from build123d import *

# Parameters (mm, degrees)
SKETCH1_W           = 900
SKETCH1_H           = 600
BOSS_EXTRUDE1_DEPTH = 5
SKETCH2_R           = 30
CUT_EXTRUDE2_DEPTH  = 10
SKETCH3_R           = 30
CUT_EXTRUDE3_DEPTH  = 10


with BuildPart() as part:
    # Sketch1 → Boss-Extrude1 (new body)
    with BuildSketch(Plane.XY):
        with Locations((25.545851528, 338.64628821)):
            Rectangle(SKETCH1_W, SKETCH1_H)
    extrude(amount=BOSS_EXTRUDE1_DEPTH)

    # Sketch2 → Cut-Extrude2 (cut)
    with BuildSketch(Plane(origin=(0, 0, 0), x_dir=(-1, 0, 0), z_dir=(0, 0, -1))):
        with Locations((-175.545851528, 535.128567936)):
            Circle(SKETCH2_R)
    extrude(amount=-CUT_EXTRUDE2_DEPTH, mode=Mode.SUBTRACT)

    # Sketch3 → Cut-Extrude3 (cut)
    with BuildSketch(Plane(origin=(0, 0, 0), x_dir=(-1, 0, 0), z_dir=(0, 0, -1))):
        with Locations((-175.545851528, 143.938114846)):
            Circle(SKETCH3_R)
    extrude(amount=-CUT_EXTRUDE3_DEPTH, mode=Mode.SUBTRACT)


solid = part.part
Can you work these out from the model? Positions are in its coordinate system, mm. Give positions to 0.01 mm unless a question says otherwise; leave off trailing zeros. Loops run counter-clockwise (first coordinate to the right, second up) from the corner with the lowest first, then second, coordinate; pieces in that order, holes last. Notation, with made-up numbers: (81, 71) -> (124, 71) arc R19 cw to (124, 84) -> close; hole circle Ø11 at (-12, -35.75). An arc over 180 degrees is marked (long way). Return JSON: item names as keys, results as strings.
Q1. I need wall thicknesses on probe 1 along X at (y, z) = (162, 2.6); probe 2 along X at (y, z) = (154, 0.85). Which ranges of each line are inside material? Lowest first, please.
Checks:
{"probe 1": "x = -424.45 to 151.59, 199.5 to 475.55", "probe 2": "x = -424.45 to 147.28, 203.81 to 475.55"}
Q2. I want a section at B-B, the plane y = 163.5. List the corners of the cut face in (x, z) for me.
Checks:
{"outline": "(-424.45, 0) -> (152.8, 0) -> (152.8, 5) -> (-424.45, 5) -> close; (198.29, 0) -> (475.55, 0) -> (475.55, 5) -> (198.29, 5) -> close"}
Q3. We'd pull the mould along X, two halves only. Please class faces 1 (the face through (19, 343, 0)), 2 (the face through (161.703, 508.513, 2.465)): released by +X, released by -X, zero draft, split by the parting line, or undercut.
Checks:
{"face 1": "zero draft", "face 2": "undercut"}
Q4. I want a section at A-A, the plane y = 521. List the corners of the cut face in (x, z) for me.
Checks:
{"outline": "(-424.45, 0) -> (149.08, 0) -> (149.08, 5) -> (-424.45, 5) -> close; (202.01, 0) -> (475.55, 0) -> (475.55, 5) -> (202.01, 5) -> close"}
